Can you work these out from the model? Positions are in its coordinate system, mm. A direction names the side the tool comes from. Give positions to 0.01 mm unless a question says otherwise; leave off trailing zeros. Loops run counter-clockwise (first coordinate to the right, second up) from the corner with the lowest first, then second, coordinate; pieces in that order, holes last. Notation, with made-up numbers: M -14.75,79.25 L 14.25,79.25 A22 cw 14.25,91.25 Z; hole C -39.75,25 d11. An arc over 180 degrees is marked long. Answer as a JSON object with one key per item and string values.
```python
from build123d import *

# Parameters (mm, degrees)
SKETCH_1_W               = 20
SKETCH_1_H               = 30
SKETCH_1_R               = 2
EXTRUDE_1_DEPTH          = 5
CUT_EXTRUDE_6_DEPTH      = 4
CUT_EXTRUDE_6_DEPTH_BACK = 4
CUT_EXTRUDE_6_START      = -15
FILLET_1_R               = 1


with BuildPart() as part:
    # 스케치1 → 보스-돌출1 (new body)
    with BuildSketch(Plane(origin=(0, 0, 0), x_dir=(1, 0, 0), z_dir=(0, 1, 0))):
        with Locations((0, 15)):
            Rectangle(SKETCH_1_W, SKETCH_1_H)
        with Locations(Location((5, 25, 0), (0, 0, 270))):
            Circle(SKETCH_1_R, mode=Mode.SUBTRACT)
        with Locations(Location((-5, 25, 0), (0, 0, 90))):
            Circle(SKETCH_1_R, mode=Mode.SUBTRACT)
        with Locations(Location((5, 5, 0), (0, 0, 270))):
            Circle(SKETCH_1_R, mode=Mode.SUBTRACT)
        with Locations(Location((-5, 5, 0), (0, 0, 90))):
            Circle(SKETCH_1_R, mode=Mode.SUBTRACT)
    extrude(amount=EXTRUDE_1_DEPTH)

    # 스케치3 → 컷-돌출6 (cut, two sides: drawn at the far end of the back side and taken through both)
    with BuildSketch(Plane(origin=(0, 0, -30), x_dir=(-1, 0, 0), z_dir=(0, 0, -1)).offset(CUT_EXTRUDE_6_START - CUT_EXTRUDE_6_DEPTH_BACK)):
        Polygon((0, 0), (-1, 1), (-2, 0), align=None)
        Polygon((1, 1), (0, 0), (2, 0), align=None)
        Polygon((-2, 0), (-3, 1), (-4, 0), align=None)
        Polygon((3, 1), (2, 0), (4, 0), align=None)
        Polygon((-4, 0), (-5, 1), (-6, 0), align=None)
        Polygon((5, 1), (4, 0), (6, 0), align=None)
        Polygon((-6, 0), (-7, 1), (-8, 0), align=None)
        Polygon((7, 1), (6, 0), (8, 0), align=None)
        Polygon((-8, 0), (-9, 1), (-10, 1), (-10, 0), align=None)
        Polygon((9, 1), (8, 0), (10, 0), (10, 1), align=None)
    extrude(amount=CUT_EXTRUDE_6_DEPTH + CUT_EXTRUDE_6_DEPTH_BACK, mode=Mode.SUBTRACT)

    # 필렛1
    fillet_1_edges = [part.edges().sort_by_distance(p)[0] for p in [
        (10, 1, -15),
        (-10, 1, -15),
    ]]
    fillet(fillet_1_edges, radius=FILLET_1_R - 0.0001)  # a hair under: the kernel refuses the full size


solid = part.part
```
1) If we mould it in two halves opening along X, with no side actions, what happens to faces 5 (the flat face through (0, 2, -30)), 6 (the flat face through (1, 0.4, -11))? For each: +X half, -X half, draft (parallel to the pull), parting line (faces both ways), or undercut.
Answer list:
{"face 5": "draft", "face 6": "undercut"}
2) Suppose I cut it at D-D, the plane y = 4.3. Write out the boundary of the cut face in (x, z).
Answer list:
{"outline": "M -10,-30 L 10,-30 L 10,0 L -10,0 Z; hole C -5,-25 d4; hole C -5,-5 d4; hole C 5,-25 d4; hole C 5,-5 d4"}
3) Please list where these lines run through material, in increasing order: line 1 along X through (y, z) = (3.4, -5); line 2 along Z through (x, y) = (-5, 2.2); line 3 along Z through (x, y) = (6.25, 0.8). Write a range as from..to.
Answer list:
{"line 1": "-10..-7, -3..3, 7..10", "line 2": "-30..-27, -23..-7, -3..0", "line 3": "-30..-26.56, -23.44..-6.56, -3.44..0"}
4) Suppose I cut it at A-A, the plane z = -25. Write out the boundary of the cut face in (x, y), and give its area (3 significant figures).
Answer list:
{"outline": "M -10,0 L -7,0 L -7,5 L -10,5 Z; M -3,0 L 3,0 L 3,5 L -3,5 Z; M 7,0 L 10,0 L 10,5 L 7,5 Z", "area": "60.0 mm^2"}
5) Suppose I cut it at B-B, the plane y = 1.6. Write out the boundary of the cut face in (x, z).
Answer list:
{"outline": "M -10,-30 L 10,-30 L 10,-19 L 9.92,-19 L 9.92,-11 L 10,-11 L 10,0 L -10,0 L -10,-11 L -9.92,-11 L -9.92,-19 L -10,-19 Z; hole C -5,-25 d4; hole C -5,-5 d4; hole C 5,-25 d4; hole C 5,-5 d4"}
6) For faces 1 (the flat face through (9.2, 0.6, -11)), 2 (the flat face through (-5, 0.4, -11)), 3 (the cylindrical face through (-5, 2, -3)), 4 (the flat face through (-9.4, 0.6, -19)), which set-ups out of +Z, -Z, +X, -X, +Y, -Y let a thin tool reach every point of the face, with its end or its side?
Answer list:
{"face 1": "+X, -Y", "face 2": "-Y", "face 3": "+Y, -Y", "face 4": "-X, -Y"}
7) Will this pin go through, and if not, where does the flat tip stop? pin 1 Ø1.5 at (x, z) = (-3.5, -15.5) entering from -Y.
Answer list:
{"pin 1": "y = 0"}
